Here's how the part is built. I have some questions about the finished solid (model axes, mm). Face numbers are marked on the shaded views. Round coordinates to 2 decimals unless told otherwise and drop trailing zeros. Write each loop counter-clockwise with the first axis right and the second up, starting at its lowest first coordinate (ties: lowest second). Pieces come first, ordered by that corner, then holes. Notation, with made-up numbers: M 73.25,22 L 119.25,22 A29 cw 119.25,47 Z; hole C 5.5,15 d7. An arc over 180 degrees is marked long. Write item = value, one per line. Start each with the question number.
(1) Will these pins go through, and if not, where does the flat tip stop? pin 1 Ø6.5 at (x, z) = (15.5, -4.5) entering from +Y; pin 2 Ø6.5 at (x, y) = (5, 68.5) entering from +Z; pin 3 Ø4 at (x, y) = (64, 4) entering from +Z; pin 4 Ø3 at (x, y) = (45.5, 17.5) entering from -Z.
(2) I want a section at D-D (y = -10.5). List the corners of the cut face in (x, z) for me, and give its area (3 significant figures).
(3) I need wall thicknesses on line 1 along Y through (x, z) = (66, 0.8); line 2 along X through (y, z) = (73.75, -4.5); line 3 along Z through (x, y) = (68, 37). Which ranges of each line are inside material? Lowest first, please.
(4) I want a section at B-B (x = 5). Give the number of separate pieces and of enclosed holes in the cut face, and give its area (3 significant figures).
(5) If we mould it in two halves opening along X, with no side actions, what happens to the marked faces 1 and 2? For each: released by +X, released by -X, zero draft, split by the parting line, or undercut.
(6) I want a section at A-A (x = 15.5). List the corners of the cut face in (y, z) for me, and give its area (3 significant figures).
```python
from build123d import *

# Parameters (mm, degrees)
SKETCH2_W           = 71
SKETCH2_H           = 73.5
BOSS_EXTRUDE1_DEPTH = 1.5
BOSS_EXTRUDE2_DEPTH = 5
SKETCH20_W          = 71
SKETCH20_H          = 1
BOSS_EXTRUDE6_DEPTH = 1.5
SKETCH12_W          = 71
SKETCH12_H          = 7
BOSS_EXTRUDE3_DEPTH = 3.5
SKETCH13_R          = 2
CUT_EXTRUDE3_DEPTH  = 75.5
SKETCH14_R          = 3.5
CUT_EXTRUDE4_DEPTH  = 2.2
SKETCH15_W          = 71
SKETCH15_H          = 1.5
BOSS_EXTRUDE4_DEPTH = 15
SKETCH16_R          = 4
SKETCH16_R_2        = 2.75
BOSS_EXTRUDE5_DEPTH = 4.5
CUT_EXTRUDE5_DEPTH  = 4
SKETCH19_R          = 2
CUT_EXTRUDE6_DEPTH  = 14.5


with BuildPart() as part:
    # Sketch2 → Boss-Extrude1 (new body)
    with BuildSketch(Plane.XY):
        with Locations((35.5, 36.75)):
            Rectangle(SKETCH2_W, SKETCH2_H)
    extrude(amount=BOSS_EXTRUDE1_DEPTH)

    # Sketch3 → Boss-Extrude2 (add)
    with BuildSketch(Plane.XY.offset(1.5)):
        Polygon((10.773502692, 68.5), (7.886751346, 73.5), (2.113248654, 73.5), (-0.773502692, 68.5), (2.113248654, 63.5), (7.886751346, 63.5), align=None)
        Polygon((63.113248654, 63.5), (60.226497308, 68.5), (63.113248654, 73.5), (68.886751346, 73.5), (71.773502692, 68.5), (68.886751346, 63.5), align=None)
        Polygon((60.226497308, 5), (63.113248654, 0), (68.886751346, 0), (71.773502692, 5), (68.886751346, 10), (63.113248654, 10), align=None)
        Polygon((7.886751346, 10), (10.773502692, 5), (7.886751346, 0), (2.113248654, 0), (-0.773502692, 5), (2.113248654, 10), align=None)
    extrude(amount=BOSS_EXTRUDE2_DEPTH)

    # Sketch20 → Boss-Extrude6 (add)
    with BuildSketch(Plane.XY.offset(1.5)):
        with Locations((35.5, 74)):
            Rectangle(SKETCH20_W, SKETCH20_H)
    extrude(amount=-BOSS_EXTRUDE6_DEPTH)

    # Sketch12 → Boss-Extrude3 (add)
    with BuildSketch(Plane.XZ.offset(-74.5)):
        with Locations((35.5, -3.5)):
            Rectangle(SKETCH12_W, SKETCH12_H)
    extrude(amount=BOSS_EXTRUDE3_DEPTH)

    # Sketch13 → Cut-Extrude3 (cut, through all)
    with BuildSketch(Plane.XZ):
        with Locations((55.5, -4.5)):
            Circle(SKETCH13_R)
        with Locations((15.5, -4.5)):
            Circle(SKETCH13_R)
    extrude(amount=-CUT_EXTRUDE3_DEPTH, mode=Mode.SUBTRACT)

    # Sketch14 → Cut-Extrude4 (cut)
    with BuildSketch(Plane(origin=(0, 74.5, 0), x_dir=(-1, 0, 0), z_dir=(0, -1, 0))):
        with Locations((-55.5, 4.5)):
            Circle(SKETCH14_R)
        with Locations((-15.5, 4.5)):
            Circle(SKETCH14_R)
    extrude(amount=CUT_EXTRUDE4_DEPTH, mode=Mode.SUBTRACT)

    # Sketch15 → Boss-Extrude4 (add)
    with BuildSketch(Plane.XZ):
        with Locations((35.5, 0.75)):
            Rectangle(SKETCH15_W, SKETCH15_H)
    extrude(amount=BOSS_EXTRUDE4_DEPTH)

    # Sketch16 → Boss-Extrude5 (add)
    with BuildSketch(Plane.XY.offset(1.5)):
        with Locations((35.5, -10.5)):
            Circle(SKETCH16_R)
        with Locations((35.5, -10.5)):
            Circle(SKETCH16_R_2, mode=Mode.SUBTRACT)
    extrude(amount=-BOSS_EXTRUDE5_DEPTH)

    # Sketch17 → Cut-Extrude5 (cut)
    with BuildSketch(Plane.XY.offset(6.5)):
        Polygon((7.309401077, 72.5), (2.690598923, 72.5), (0.381197846, 68.5), (2.690598923, 64.5), (7.309401077, 64.5), (9.618802154, 68.5), align=None)
        Polygon((68.309401077, 72.5), (63.690598923, 72.5), (61.381197846, 68.5), (63.690598923, 64.5), (68.309401077, 64.5), (70.618802154, 68.5), align=None)
        Polygon((68.309401077, 9), (63.690598923, 9), (61.381197846, 5), (63.690598923, 1), (68.309401077, 1), (70.618802154, 5), align=None)
        Polygon((7.309401077, 9), (2.690598923, 9), (0.381197846, 5), (2.690598923, 1), (7.309401077, 1), (9.618802154, 5), align=None)
    extrude(amount=-CUT_EXTRUDE5_DEPTH, mode=Mode.SUBTRACT)

    # Sketch19 → Cut-Extrude6 (cut, through all)
    with BuildSketch(Plane.XY.offset(6.5)):
        with Locations((5, 68.5)):
            Circle(SKETCH19_R)
        with Locations((66, 68.5)):
            Circle(SKETCH19_R)
        with Locations((5, 5)):
            Circle(SKETCH19_R)
        with Locations((66, 5)):
            Circle(SKETCH19_R)
    extrude(amount=-CUT_EXTRUDE6_DEPTH, mode=Mode.SUBTRACT)


solid = part.part
```
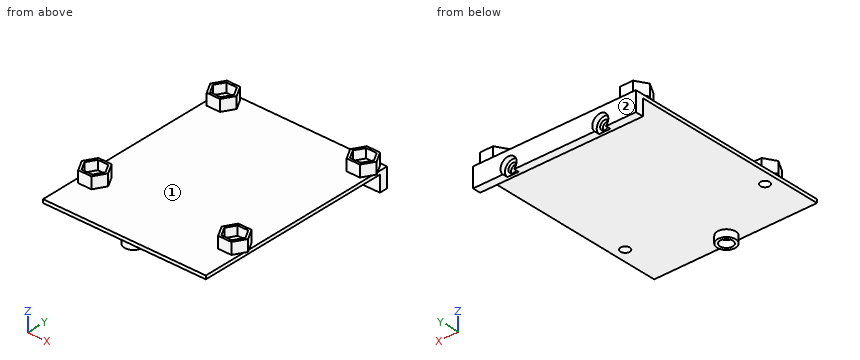
Returned:
q1.pin_1 = 72.3
q1.pin_2 = 2.5
q1.pin_3 = 6.5
q1.pin_4 = 0
q2.outline = M 0,0 L 31.5,0 L 31.5,-3 L 32.75,-3 L 32.75,0 L 38.25,0 L 38.25,-3 L 39.5,-3 L 39.5,0 L 71,0 L 71,1.5 L 0,1.5 Z
q2.area = 114 mm²
q3.line_1 = -15 to 3, 7 to 66.5, 70.5 to 74.5
q3.line_2 = 0 to 12, 19 to 52, 59 to 71
q3.line_3 = 0 to 1.5
q4.separate_pieces = 3
q4.enclosed_holes = 0
q4.area = 175 mm²
q5.face_1 = undercut
q5.face_2 = zero draft
q6.outline = M -15,0 L 71,0 L 71,-2.5 L 72.3,-2.5 L 72.3,-1 L 74.5,-1 L 74.5,1.5 L -15,1.5 Z; M 71,-7 L 72.3,-7 L 72.3,-6.5 L 71,-6.5 Z
q6.area = 140 mm²
